Autodesk Inventor part; units mm, degrees
ref_plane "YZ Plane" through (0, 0, 0) normal (1, 0, 0) x (0, 1, 0)
ref_plane "XZ Plane" through (0, 0, 0) normal (0, 1, 0) x (-1, 0, 0)
ref_plane "XY Plane" through (0, 0, 0) normal (0, 0, 1) x (1, 0, 0)
sketch "Skizze1" plane through (0, 0, 0) normal (0, 0, 1) x (1, 0, 0)
  line L0 (-53, -3.85) -> (53, -3.85)
  line L1 (53, -3.85) -> (53, 3.85)
  line L2 (53, 3.85) -> (-53, 3.85)
  line L3 (-53, 3.85) -> (-53, -3.85)
  line L4 (-53, -3.85) -> (53, 3.85) construction
  line L5 (53, -3.85) -> (-53, 3.85) construction
  point P0 (0, 0)
  dimension "d0" = 7.7
  dimension "d1" = 106
extrude "Extrusion1" add sketch "Skizze1" along normal blind 3.8
sketch "Skizze2" plane through (0, 0, 3.8) normal (0, 0, 1) x (1, 0, 0)
  line L0 (53, 3.85) -> (-53, 3.85) construction
  line L1 (50, 3.85) -> (50, -3.85) construction
  line L2 (-53, -3.85) -> (53, -3.85) construction
  line L3 (53, -3.85) -> (53, 3.85) construction
  circle A0 centre (50, 0) radius 1.85
  line L4 (0, 3.85) -> (0, -3.85) construction
  circle A1 centre (-50, 0) radius 1.85
  point P0 (0, 0)
  dimension "d4" = 3
  dimension "d5" = 3.7
extrude "Extrusion2" cut sketch "Skizze2" against normal through all
properties part number "3_3D-Druck"
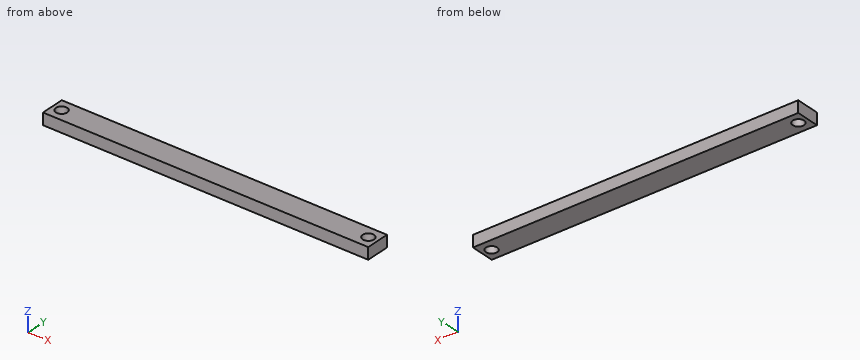
Model file for the job. Use its own axes, mm. Coordinates: 2 decimals unless noted, no trailing zeros. Write each loop counter-clockwise with the first axis right and the second up, starting at its lowest first coordinate (ties: lowest second). Pieces come first, ordered by that corner, then holes. Notation, with made-up numbers: (-1, 60) - (27, 60) arc R16 ccw to (27, 75) - close; hole circle Ø10 at (49, -37.5). An arc over 180 degrees is marked (long way). Write each question's results on one line, items separated by ' | '. Start each with the question number.
1) Cut at C-C (y = 0). Write the cut outline in (x, z), then the cut area to 3 significant figures.
2) Probe line 1 along X through (y, z) = (0.25, 2.55); line 2 along Y through (x, z) = (-50, 1.8); line 3 along X through (y, z) = (-1.25, 1.5). List the from-to ranges inside material, lowest first. Write a range as from..to.
3) Flat gauge pin, fed straight in: P1, Ø3.5, axis at x = 50, y = 0, coming from the +Z side. Where does the tip first touch, or does it go through?
4) Cut at B-B (z = 0.6). Write the cut outline in (x, y).
5) Cut at A-A (x = -50). Write the cut outline in (y, z), then the cut area to 3 significant figures.
Returned:
1) outline: (-53, 0) - (-51.85, 0) - (-51.85, 3.8) - (-53, 3.8) - close; (-48.15, 0) - (48.15, 0) - (48.15, 3.8) - (-48.15, 3.8) - close; (51.85, 0) - (53, 0) - (53, 3.8) - (51.85, 3.8) - close | area: 375 mm^2
2) line 1: -53..-51.83, -48.17..48.17, 51.83..53 | line 2: -3.85..-1.85, 1.85..3.85 | line 3: -53..-51.36, -48.64..48.64, 51.36..53
3) P1: through
4) outline: (-53, -3.85) - (53, -3.85) - (53, 3.85) - (-53, 3.85) - close; hole circle Ø3.7 at (-50, 0); hole circle Ø3.7 at (50, 0)
5) outline: (-3.85, 0) - (-1.85, 0) - (-1.85, 3.8) - (-3.85, 3.8) - close; (1.85, 0) - (3.85, 0) - (3.85, 3.8) - (1.85, 3.8) - close | area: 15.2 mm^2
